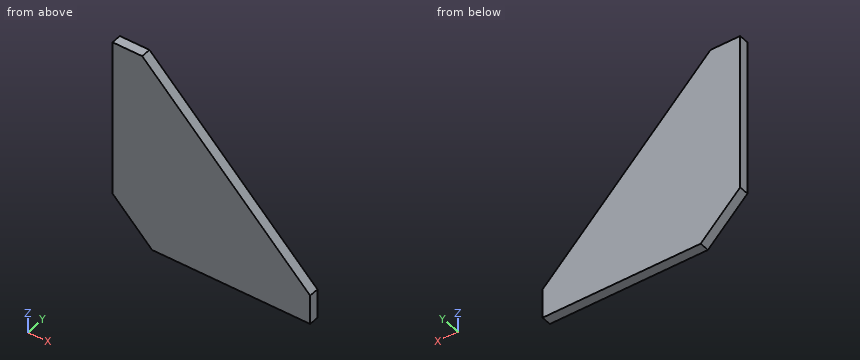
from build123d import *

# Parameters (mm, degrees)
PAD_DEPTH = 5


with BuildPart() as part:
    # Sketch → Pad (new body, symmetric)
    with BuildSketch(Plane.XZ):
        Polygon((40, 0), (200, 0), (200, 30), (30, 200), (0, 200), (0, 40), align=None)
    extrude(amount=PAD_DEPTH, both=True)


solid = part.part
Design review of the part built by this model. Coordinates are the model's own, in mm. Give positions to 0.01 mm unless a question says otherwise; leave off trailing zeros. Loops run counter-clockwise (first coordinate to the right, second up) from the corner with the lowest first, then second, coordinate; pieces in that order, holes last. Notation, with made-up numbers: (-15.5, 48) - (21.5, 48) arc R16 cw to (21.5, 76) - close; hole circle Ø1 at (43, 5). An arc over 180 degrees is marked (long way). Write item = value, one per line.
1) Take a section at C-C on x = 46. State the section outline as (y, z) points, and give its area (3 significant figures).
Result sheet:
outline = (-5, 0) - (5, 0) - (5, 184) - (-5, 184) - close
area = 1,840 mm2
2) Take a section at B-B on y = 2.5. State the section outline as (x, z) points, and give its area (4 significant figures).
Result sheet:
outline = (0, 40) - (40, 0) - (200, 0) - (200, 30) - (30, 200) - (0, 200) - close
area = 24,750 mm2
3) To check wall thickness, follow line 1 (X direction, y = 0.75, z = 104.5); line 2 (Z direction, x = 92, y = 1.75); line 3 (Z direction, x = 118, y = -4.25). State the ranges of each line that lie inside material, in increasing order.
Result sheet:
line_1 = 0 to 125.5
line_2 = 0 to 138
line_3 = 0 to 112
4) Clearance check with flat-ended pins moving along their axes: pin 1 Ø4 at (x, y) = (48.5, -3.5) entering from +Z; pin 2 Ø1.5 at (y, z) = (1.5, 121.5) entering from +X. State where each tip first meets the part, or that it passes through.
Result sheet:
pin_1 = 183.5
pin_2 = 109.25
5) Take a section at A-A on z = 93. State the section outline as (x, y) points.
Result sheet:
outline = (0, -5) - (137, -5) - (137, 5) - (0, 5) - close
